CAD build for the part. Positions are in the model's coordinates, mm. Round coordinates to 2 decimals unless told otherwise and drop trailing zeros. Loops run counter-clockwise (first coordinate to the right, second up) from the corner with the lowest first, then second, coordinate; pieces in that order, holes last. Notation, with made-up numbers: M -37.75,-7 L -28.75,-7 A8 cw -28.75,8 Z; hole C 10,48.5 d3. An arc over 180 degrees is marked long. Use a Markdown table: item, result. Add a question column.
(1) Two-plate mould, pull along Y, no slides. Class faces 1 (the face through (7.62, 31, 2)), 2 (the face through (-63, 69.431, -29)), 3 (the face through (-59, -62.582, 0)): released by +Y, released by -Y, zero draft, split by the parting line, or undercut.
(2) Flat gauge pin, fed straight in: P1, Ø10, axis at y = -1, z = 22.5, coming from the -X side. Where does the tip first touch, or does it go through?
(3) Band-saw the part on A-A, the plane x = -116.5. Write the cut outline in (y, z), and give its area (3 significant figures).
(4) Band-saw the part on B-B, the plane y = -24.5. Write the cut outline in (x, z), and give its area (3 significant figures).
(5) Wall check: L1, parallel to Y at x = -118, z = 42; L2, parallel to Z at x = -98, y = 70.5; L3, parallel to X at y = -17, z = 44.5. Give the ranges that are in metal, low to high.
(6) Band-saw the part on C-C, the plane z = 11.5. Write the cut outline in (x, y), and give its area (3 significant figures).
from build123d import *

# Parameters (mm, degrees)
F0_W     = 190.5
F0_H     = 127
F1_DEPTH = 7.62
F2_W     = 7.7119544148
F2_H     = 7.6466050446
F2_W_2   = 175.0760897994
F2_H_2   = 111.7067933083
F2_W_3   = 7.7119557858
F2_H_3   = 7.6466016471
F3_DEPTH = 127
F4_W     = 7.6109431684
F4_H     = 52.9533312656
F4_H_2   = 7.6109394431
F4_W_2   = 48.9413635805
F4_W_3   = 8.3309542388
F4_W_4   = 59.4186419621
F5_DEPTH = 127


with BuildPart() as f1:
    # F0 (on Right) → F1 (new body)
    with BuildSketch(Plane.YZ):
        with Locations((32.6675430536, 0.8675659299)):
            Rectangle(F0_W, F0_H)
    extrude(amount=F1_DEPTH)

    # F2 (on face) → F3 (join)
    with BuildSketch(Plane(origin=(0, 0, 0), x_dir=(0, -1, 0), z_dir=(-1, 0, 0))):
        with Locations((-124.0615658462, 60.5442634076)):
            Rectangle(F2_W, F2_H)
        with Locations((-32.6675437391, 60.5442634076)):
            Rectangle(F2_W_2, F2_H)
        with Locations((-124.0615658462, 0.8675642312)):
            Rectangle(F2_W, F2_H_2)
        with Locations((58.7264790535, 60.5442634076)):
            Rectangle(F2_W_3, F2_H)
        with Locations((-124.0615658462, -58.8091332465)):
            Rectangle(F2_W, F2_H_3)
        with Locations((58.7264790535, 0.8675642312)):
            Rectangle(F2_W_3, F2_H_2)
        with Locations((-32.6675437391, -58.8091332465)):
            Rectangle(F2_W_2, F2_H_3)
        with Locations((58.7264790535, -58.8091332465)):
            Rectangle(F2_W_3, F2_H_3)
    extrude(amount=F3_DEPTH)

    # F4 (on face) → F5 (join)
    with BuildSketch(Plane(origin=(0, 0, 0), x_dir=(0, -1, 0), z_dir=(-1, 0, 0))):
        with Locations((-65.625930205, 30.2442952525)):
            Rectangle(F4_W, F4_H)
        with Locations((-65.625930205, -0.0378401019)):
            Rectangle(F4_W, F4_H_2)
        Polygon((-69.4314017892, -3.8433098234), (-69.4314017892, 3.7676296197), (-110.6796637177, 3.7676296197), (-120.2055886388, 3.7676296197), (-120.2055886388, 0), (-120.2055886388, -3.8433098234), align=None)
        Polygon((-61.8204586208, -3.8433098234), (-69.4314017892, -3.8433098234), (-69.4314017892, -24.8306896538), (-69.4314017892, -54.985832423), (-61.8204586208, -54.985832423), align=None)
        with Locations((-37.3497768305, -0.0378401019)):
            Rectangle(F4_W_2, F4_H_2)
        with Locations((-8.7136179209, -0.0378401019)):
            Rectangle(F4_W_3, F4_H_2)
        with Locations((-8.7136179209, 30.2442952525)):
            Rectangle(F4_W_3, F4_H)
        Polygon((-4.5481408015, -3.8433098234), (-12.8790950403, -3.8433098234), (-12.8790950403, -54.985832423), (-4.5481408015, -54.985832423), (-4.5481408015, -8.6574442685), align=None)
        with Locations((25.1611801796, -0.0378401019)):
            Rectangle(F4_W_4, F4_H_2)
    extrude(amount=F5_DEPTH)


solid = f1.part
Return value:
| question | item | result |
|---|---|---|
| 1 | face 1 | zero draft |
| 1 | face 2 | undercut |
| 1 | face 3 | released by -Y |
| 2 | P1 | x = 0 |
| 3 | outline | M -62.58,-62.63 L 127.92,-62.63 L 127.92,64.37 L -62.58,64.37 Z; hole M -54.87,-54.99 L 4.55,-54.99 L 4.55,-3.84 L -54.87,-3.84 Z; hole M -54.87,3.77 L 4.55,3.77 L 4.55,56.72 L -54.87,56.72 Z; hole M 12.88,-54.99 L 61.82,-54.99 L 61.82,-3.84 L 12.88,-3.84 Z; hole M 12.88,3.77 L 61.82,3.77 L 61.82,56.72 L 12.88,56.72 Z; hole M 69.43,-54.99 L 120.21,-54.99 L 120.21,-3.84 L 69.43,-3.84 Z; hole M 69.43,3.77 L 120.21,3.77 L 120.21,56.72 L 69.43,56.72 Z |
| 3 | area | 7,630 mm^2 |
| 4 | outline | M -127,-62.63 L 7.62,-62.63 L 7.62,64.37 L -127,64.37 L -127,56.72 L 0,56.72 L 0,3.77 L -127,3.77 L -127,-3.84 L 0,-3.84 L 0,-54.99 L -127,-54.99 Z |
| 4 | area | 3,880 mm^2 |
| 5 | L1 | -62.58 to -54.87, 4.55 to 12.88, 61.82 to 69.43, 120.21 to 127.92 |
| 5 | L2 | -62.63 to -54.99, -3.84 to 3.77, 56.72 to 64.37 |
| 5 | L3 | 0 to 7.62 |
| 6 | outline | M -127,-62.58 L 7.62,-62.58 L 7.62,127.92 L -127,127.92 L -127,120.21 L 0,120.21 L 0,69.43 L -127,69.43 L -127,61.82 L 0,61.82 L 0,12.88 L -127,12.88 L -127,4.55 L 0,4.55 L 0,-54.87 L -127,-54.87 Z |
| 6 | area | 5,440 mm^2 |
